Input: dimensioned drawing with shaded views. Units: mm. Origin: part minimum x, y, z. Round coordinates to 2 decimals unless told otherwise and drop trailing zeros. Write each loop counter-clockwise with the first axis right and the second up, starting at its lowest first coordinate (ties: lowest second). Pieces come first, ordered by that corner, then holes. Notation, with made-up numbers: (-38.75, 25.5) - (-30.75, 25.5) arc R20 cw to (-30.75, 34.5) - close; hole circle Ø5 at (-4.5, 48). An arc over 180 degrees is marked (long way). Write item = value, one per line. Start each with the question number.
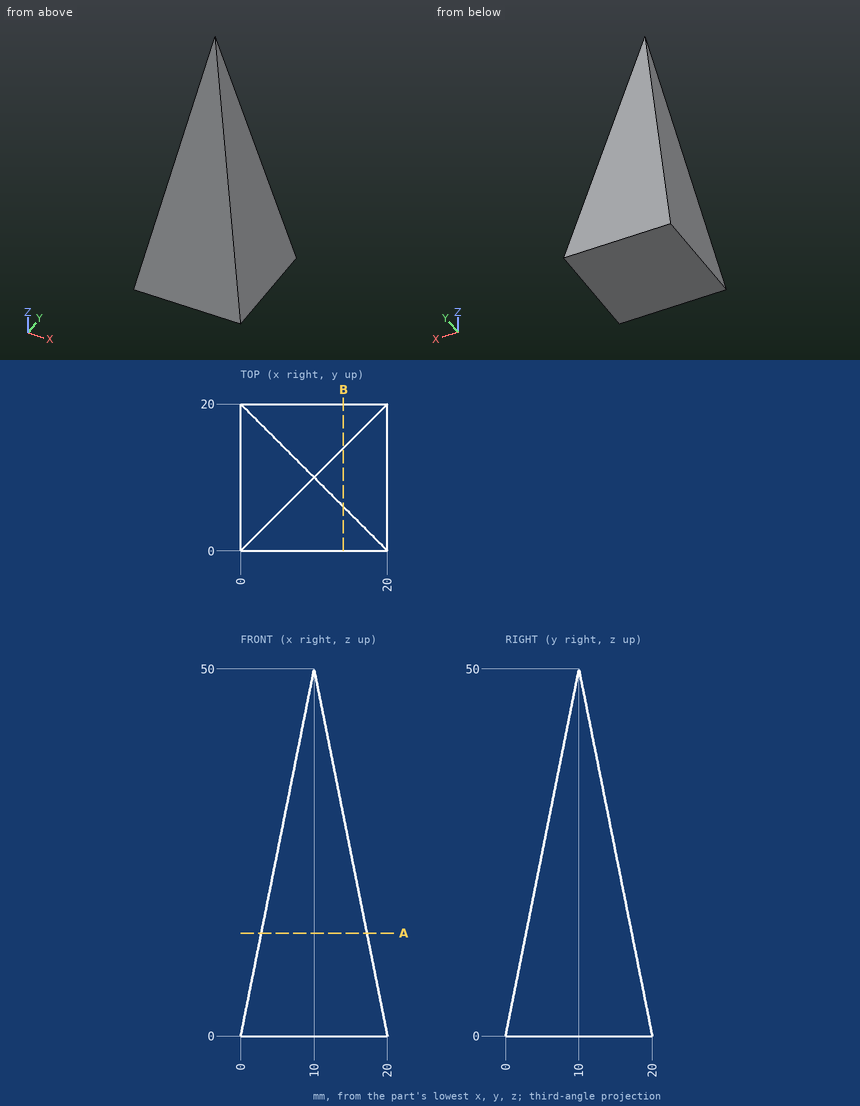
(1) Section B-B (x = 14). Return the cut outline in (y, z), plus the area to 3 significant figures.
(2) Ray query, L1, parallel to Y at x = 10.75, z = 39; L2, parallel to X at y = 3, z = 7.5; L3, parallel to X at y = 13.75, z = 9. Return the intervals inside material, ascending. Write a range as from..to.
(3) Section A-A (z = 14). Return the cut outline in (x, y), plus the area to 3 significant figures.
(4) Contact query for flat-ended pins moving along their axis: P1, Ø12, axis at x = 5, z = 23.5, coming from the -Y side; P2, Ø12, axis at x = 7.5, z = 44.5, coming from the -Y side; P3, Ø6, axis at x = 15.5, z = 19.5, coming from the -Y side. Output: stop coordinate, or through.
Solution:
q1.outline = (0, 0) - (20, 0) - (14, 30) - (6, 30) - close
q1.area = 420 mm^2
q2.L1 = 7.8..12.2
q2.L2 = 1.5..18.5
q2.L3 = 1.8..18.2
q3.outline = (2.8, 2.8) - (17.2, 2.8) - (17.2, 17.2) - (2.8, 17.2) - close
q3.area = 207 mm^2
q4.P1 = 3.5
q4.P2 = 7.7
q4.P3 = 3.3
